Autodesk Inventor part; units mm, degrees
ref_plane "Work Plane1" through (-3, 0, 0) normal (1, 0, 0) x (0, 1, 0)
ref_plane "Work Plane2" through (0, 9, 0) normal (0, 1, 0) x (-1, 0, 0)
ref_plane "XY Plane" through (0, 0, 0) normal (0, 0, 1) x (1, 0, 0)
sketch "Sketch1" plane through (0, 0, 0) normal (0, 0, 1) x (1, 0, 0)
  circle A0 centre (0, 0) radius 3
  line L0 (74, 5) -> (74, -5) construction
  point P0 (74, 0)
  dimension "d0" = 6
  dimension "d1" = 148
  dimension "d2" = 10
revolve "Revolution1" add sketch "Sketch1" angle 360 about axis through (74, 5, 0) along (0, -1, 0)
ref_plane "Work Plane1" through (-3, 0, 0) normal (1, 0, 0) x (0, 1, 0)
sketch "Sketch2" plane through (-3, 0, 0) normal (1, 0, 0) x (0, 1, 0)
  circle A0 centre (6, 0) radius 3
  line L0 (6, 3) -> (0, 3)
  line L1 (0, 3) -> (0, -3)
  line L2 (0, -3) -> (6, -3)
  point P0 (0, 0)
  dimension "d5" = 6
  dimension "d6" = 6
  dimension "d7" = 6
  dimension "d8" = 6
extrude "Extrusion1" add sketch "Sketch2" along normal blind 6
sketch "Sketch3" plane through (3, 0, 0) normal (1, 0, 0) x (0, 0, -1)
  arc A0 (3, 6) -> (-3, 6) centre (0, 6) ccw
  circle A1 centre (0, 6) radius 3
  dimension "d11" = 6
extrude "Extrusion2" add sketch "Sketch3" along normal blind 26
pattern_circular "Circular Pattern1" count 3 over 360 about axis through (74, 0, 0) along (0, 1, 0) of "Extrusion1", "Extrusion2"
ref_plane "Work Plane2" through (0, 9, 0) normal (0, 1, 0) x (-1, 0, 0)
sketch "Sketch4" plane through (0, 9, 0) normal (0, 1, 0) x (-1, 0, 0)
  circle A0 centre (-74, 0) radius 45.5
  point P0 (0, 0)
  dimension "d18" = 91
  dimension "d19" = 74
extrude "Extrusion3" cut sketch "Sketch4" against normal blind 26
properties part number "Kern" material "Silicon Nitride"
CAD build for the part. Positions are in the model's coordinates, mm. A direction names the side the tool comes from. Coordinates: 2 decimals unless noted, no trailing zeros. Use a Markdown table: item, result. Add a question column.
(1) Pull direction X, two halves, no side cores. Call faces 3 (the face through (-3, 4, 0)), 4 (the face through (109.536, 2.291, 61.467)), 5 (the face through (28.5, 6, 0)), 6 (the face through (3, 2, 0)): +X half, -X half, draft (parallel to the pull), parting line (faces both ways), or undercut.
(2) Drill centre lines: line 1 along Z through (x, y) = (110.5, 2.25); line 2 along X through (y, z) = (0.5, 32); line 3 along Z through (x, y) = (88.5, 2). Where is each one in solid material? Low to high. Write a range as [from, to].
(3) Which spindle directions (+Z, -Z, +X, -X, +Y, -Y) get a long thin tool onto all of the face, cutting with end or side? Do faces 1 (the face through (96.714, 6.042, 39.425)), 2 (the face through (113.62, 4.29, -62.62)). Say none if no direction does.
(4) Saw through at A-A (x = 96). Count the separate pieces of the cut face and the enclosed holes in it, then the cut area to 3 significant figures.
(5) Flat gauge pins, fed straight in: pin 1 (1.5 mm diameter, centred on x = 74.5, y = -1, fed in from +Z); pin 2 (1.2 mm diameter, centred on x = 114, z = -65.5, fed in from -Y); pin 3 (1.8 mm diameter, centred on x = 0.5, y = 4, fed in from +Z). Where does each tip first touch, or does it go through?
Solved:
| question | item | result |
|---|---|---|
| 1 | face 3 | -X half |
| 1 | face 4 | undercut |
| 1 | face 5 | +X half |
| 1 | face 6 | undercut |
| 2 | line 1 | z = [-67.84, -60.91], [60.91, 67.84] |
| 2 | line 2 | x = [4.01, 10.57], [137.43, 143.99] |
| 2 | line 3 | z = [-74.84, -70.28], [70.28, 74.84] |
| 3 | face 1 | -X, +Y, -Y |
| 3 | face 2 | +Y |
| 4 | separate pieces | 4 |
| 4 | enclosed holes | 0 |
| 4 | area | 95.4 mm² |
| 5 | pin 1 | stops at z = 76.99 |
| 5 | pin 2 | stops at y = -2.09 |
| 5 | pin 3 | stops at z = 3 |
